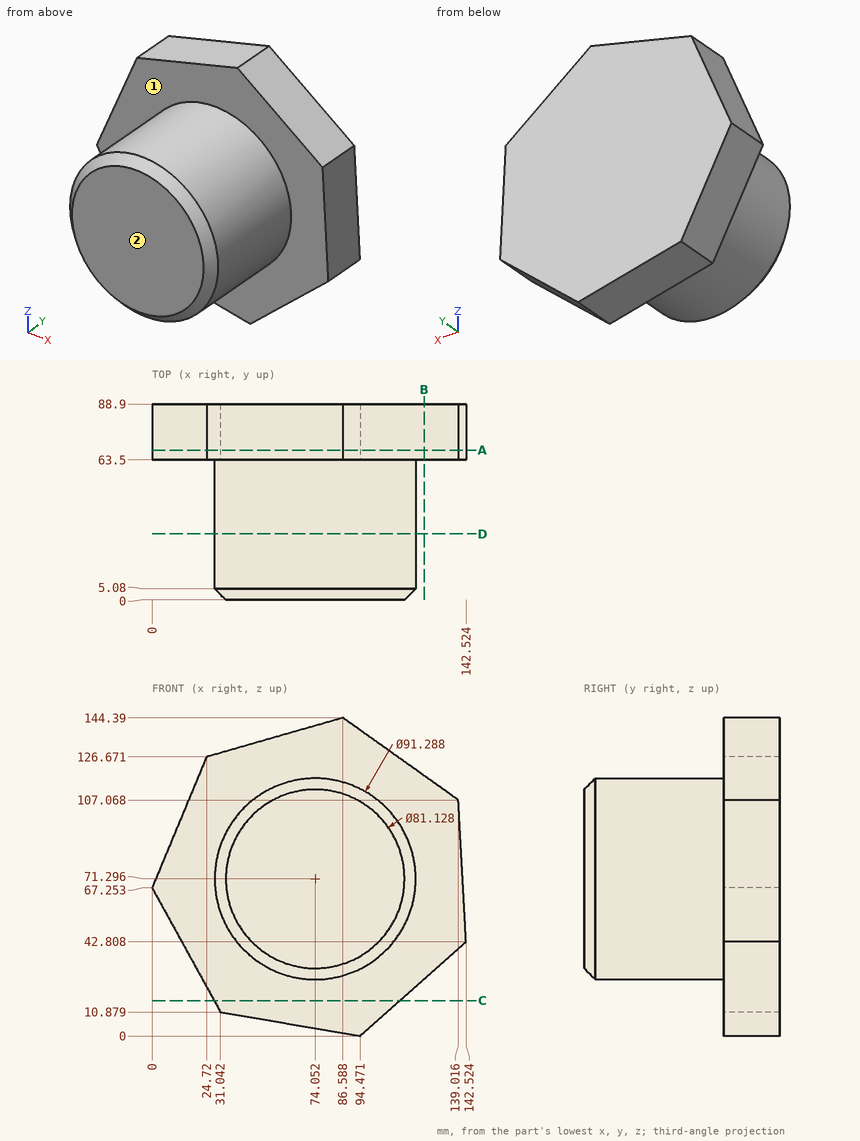
Verification items for this drawing (mm, ordinates from the low corner). A direction names the side the tool comes from. Round coordinates to 2 decimals unless told otherwise and drop trailing zeros. Order: outer loops, then holes, each group sorted by start corner. A loop starts at its lowest first (then second) coordinate and runs counter-clockwise, first axis right, second up. Notation, with made-up numbers: M 84,35.25 L 115,35.25 A15 cw 115,57.25 Z; hole C 15.5,83 d2. An arc over 180 degrees is marked long. Answer in a Markdown table with one row per item. Add a question column.
Item 1: Set-up check for the marked faces 1 and 2: record each of +Z, -Z, +X, -X, +Y, -Y from which the full face is reachable in a straight line by a thin tool's end or side.
Item 2: Sectioned sample at B-B, the plane x = 123.5. Enter the section's corners in (y, z).
Item 3: Sectioned sample at A-A, the plane y = 68. Enter the section's corners in (x, z) (1 decimal).
Item 4: Sectioned sample at C-C, the plane z = 16. Enter the section's corners in (x, y), plus the area to 3 significant figures.
Item 5: Material ranges on L1, parallel to Y at x = 63, z = 11.5; L2, parallel to X at y = 31, z = 75 (1 decimal); L3, parallel to Z at x = 104.5, y = 67 (1 decimal), recorded low to high. Write a range as [from, to].
Item 6: Sectioned sample at D-D, the plane y = 30. Enter the section's corners in (x, z) (1 decimal), plus the area to 4 significant figures.
Item 7: Depth check by flat-ended pin: pin 1 Ø2 at (x, y) = (100, 71) entering from +Z (1 decimal); pin 2 Ø8 at (y, z) = (63, 87) entering from -X (1 decimal); pin 3 Ø5 at (y, z) = (34, 77) entering from +X. Enter the tip coordinate at first touch or a pass-through.
Filled in:
| question | item | result |
|---|---|---|
| 1 | face 1 | -Y |
| 1 | face 2 | +Z, -Z, +X, -X, -Y |
| 2 | outline | M 63.5,25.86 L 88.9,25.86 L 88.9,118.11 L 63.5,118.11 Z |
| 3 | outline | M 0,67.3 L 31,10.9 L 94.5,0 L 142.5,42.8 L 139,107.1 L 86.6,144.4 L 24.7,126.7 Z |
| 4 | outline | M 28.22,63.5 L 112.43,63.5 L 112.43,88.9 L 28.22,88.9 Z |
| 4 | area | 2,140 mm² |
| 5 | L1 | y = [63.5, 88.9] |
| 5 | L2 | x = [28.6, 119.5] |
| 5 | L3 | z = [8.9, 131.6] |
| 6 | outline | C 74.1,71.3 d91.3 |
| 6 | area | 6,545 mm² |
| 7 | pin 1 | stops at z = 135.6 |
| 7 | pin 2 | stops at x = 6.6 |
| 7 | pin 3 | stops at x = 119.58 |
